from build123d import *

# Parameters (mm, degrees)
BOSS_EXTRUDE1_DEPTH = 10
CUT_EXTRUDE1_DEPTH  = 42.158231255
FILLET1_R           = 3
BOSS_EXTRUDE2_DEPTH = 3.5
SKETCH4_W           = 8
SKETCH4_H           = 2.5
BOSS_EXTRUDE3_DEPTH = 5
CIRPATTERN1_COUNT   = 2
CIRPATTERN1_ANGLE   = 180


with BuildPart() as part:
    # Sketch1 → Boss-Extrude1 (new, symmetric)
    with BuildSketch(Plane(origin=(0, 0, 0), x_dir=(1, 0, 0), z_dir=(0, 1, 0))):
        with BuildLine():
            Line((-9, 0), (9.75, 0))
            ThreePointArc((9.75, 0), (13.639087297, -1.610912703), (15.25, -5.5))
            Line((15.25, -5.5), (15.25, -9.5))
            ThreePointArc((15.25, -9.5), (16.128679656, -11.621320344), (18.25, -12.5))
            Line((18.25, -12.5), (37, -12.5))
            Line((37, -12.5), (37, -15))
            Line((37, -15), (18.25, -15))
            ThreePointArc((18.25, -15), (14.360912703, -13.389087297), (12.75, -9.5))
            Line((12.75, -9.5), (12.75, -5.5))
            ThreePointArc((12.75, -5.5), (11.871320344, -3.378679656), (9.75, -2.5))
            Line((9.75, -2.5), (-9, -2.5))
            Line((-9, -2.5), (-9, 0))
        make_face()
    extrude(amount=BOSS_EXTRUDE1_DEPTH, both=True)

    # Sketch2 → Cut-Extrude1 (cut, through all)
    with BuildSketch(Plane.XY):
        with BuildLine():
            Line((-2.75, 0), (-2.75, -10))
            Line((-2.75, -10), (2.75, -10))
            Line((2.75, -10), (2.75, 0))
            ThreePointArc((2.75, 0), (0, 2.75), (-2.75, 0))
        make_face()
        with BuildLine():
            Line((25.25, 0), (25.25, -10))
            Line((25.25, -10), (30.75, -10))
            Line((30.75, -10), (30.75, 0))
            ThreePointArc((30.75, 0), (28, 2.75), (25.25, 0))
        make_face()
    extrude(amount=CUT_EXTRUDE1_DEPTH, mode=Mode.SUBTRACT)

    # Fillet1
    fillet1_edges = [part.edges().sort_by_distance(p)[0] for p in [
        (37, -10, 13.75),
        (-9, -10, 1.25),
        (37, 10, 13.75),
        (2.75, -10, 1.25),
        (-2.75, -10, 1.25),
        (-9, 10, 1.25),
        (25.25, -10, 13.75),
        (30.75, -10, 13.75),
    ]]
    fillet(fillet1_edges, radius=FILLET1_R)

    # Sketch3 → Boss-Extrude2 (add)
    with BuildSketch(Plane.XY.offset(2.5)):
        Polygon((0, 4.618802154), (-4, 2.309401077), (-4, -2.309401077), (0, -4.618802154), (4, -2.309401077), (4, 2.309401077), align=None)
    boss_extrude2 = extrude(amount=BOSS_EXTRUDE2_DEPTH)

    # Sketch4 → Revolve1 (revolve)
    with BuildSketch(Plane(origin=(0, 0, 0), x_dir=(0, 0, -1), z_dir=(1, 0, 0))):
        with Locations((1.5, 1.25)):
            Rectangle(SKETCH4_W, SKETCH4_H)
    revolve1 = revolve(axis=Axis((0, 0, -5.5), (0, 0, 1)))

    # Sketch5 → Cut-Revolve1 (revolve, cut)
    with BuildSketch(Plane(origin=(0, 0, 0), x_dir=(0, 0, -1), z_dir=(1, 0, 0))):
        Polygon((-2.5, 4.618802154), (-2.5, 4), (-2.85726559, 4.618802154), align=None)
        Polygon((-5.64273441, 4.618802154), (-6, 4.618802154), (-6, 4), align=None)
    cut_revolve1 = revolve(axis=Axis((0, 0, 2.5), (0, 0, 1)), mode=Mode.SUBTRACT)

    # Sketch6 → Boss-Extrude3 (add, symmetric)
    with BuildSketch(Plane(origin=(0, 0, 0), x_dir=(0, 0, -1), z_dir=(1, 0, 0))):
        with BuildLine():
            Line((5.172072931, 2.989575498), (2.36192258, 4.957263957))
            ThreePointArc((2.36192258, 4.957263957), (2.123797819, 4.972871479), (2, 4.768858987))
            Line((2, 4.768858987), (2, 2.9))
            Line((2, 2.9), (1.4, 2.9))
            ThreePointArc((1.4, 2.9), (1.258578644, 2.841421356), (1.2, 2.7))
            Line((1.2, 2.7), (1.2, -2.7))
            ThreePointArc((1.2, -2.7), (1.258578644, -2.841421356), (1.4, -2.9))
            Line((1.4, -2.9), (2, -2.9))
            Line((2, -2.9), (2, -4.768858987))
            ThreePointArc((2, -4.768858987), (2.123797819, -4.972871479), (2.36192258, -4.957263957))
            Line((2.36192258, -4.957263957), (5.172072931, -2.989575498))
            ThreePointArc((5.172072931, -2.989575498), (5.26610325, -2.882354469), (5.3, -2.743829885))
            Line((5.3, -2.743829885), (5.3, 2.743829885))
            ThreePointArc((5.3, 2.743829885), (5.26610325, 2.882354469), (5.172072931, 2.989575498))
        make_face()
    boss_extrude3 = extrude(amount=BOSS_EXTRUDE3_DEPTH, both=True)

    # CirPattern1: Boss-Extrude2, Revolve1, Cut-Revolve1, Boss-Extrude3 ×2 about axis
    cirpattern1_axis = Axis((14, 11, 7.5), (0, -1, 0))
    add([boss_extrude2.rotate(cirpattern1_axis, i * CIRPATTERN1_ANGLE / (CIRPATTERN1_COUNT - 1)) for i in range(1, CIRPATTERN1_COUNT)])
    add([revolve1.rotate(cirpattern1_axis, i * CIRPATTERN1_ANGLE / (CIRPATTERN1_COUNT - 1)) for i in range(1, CIRPATTERN1_COUNT)])
    add([cut_revolve1.rotate(cirpattern1_axis, i * CIRPATTERN1_ANGLE / (CIRPATTERN1_COUNT - 1)) for i in range(1, CIRPATTERN1_COUNT)], mode=Mode.SUBTRACT)
    add([boss_extrude3.rotate(cirpattern1_axis, i * CIRPATTERN1_ANGLE / (CIRPATTERN1_COUNT - 1)) for i in range(1, CIRPATTERN1_COUNT)])


solid = part.part
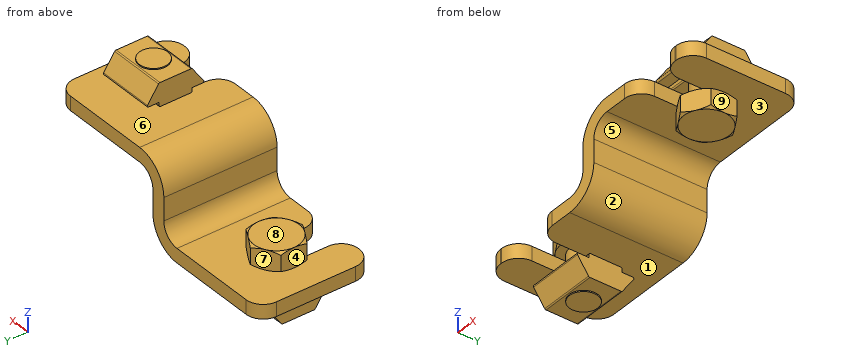
Design review of the part built by this model. Coordinates are the model's own, in mm. Face numbers are marked on the shaded views. A direction names the side the tool comes from. Give positions to 0.01 mm unless a question says otherwise; leave off trailing zeros. Order: outer loops, then holes, each group sorted by start corner. A loop starts at its lowest first (then second) coordinate and runs counter-clockwise, first axis right, second up. Notation, with made-up numbers: (-16, 88.5) - (42, 88.5) arc R32 ccw to (42, 124.5) - close; hole circle Ø2 at (88.25, -14.5). An arc over 180 degrees is marked (long way). Use CSV: the item, a comma, the result in double quotes. Start each with the question number.
Q1. Take a section at A-A (z = 11.5). State the section outline as (x, y) points.
Q2. Machinability: for the marked faces 5, 6, 7, 8 and 9, which of the approach directions +Z, -Z, +X, -X, +Y, -Y give a long, thin tool a straight path to every point of the face, cutting with its end or side? Answer none if there is none.
Q3. Draft analysis for pull direction X (two halves, no side actions). For the marked faces 1, 2, 3 and 4, state which applies: pulls with the +X half, pulls with the -X half, needs draft (parallel to the pull), parting line crosses it, or undercut.
Q4. For P1, Ø3, axis at y = -4.5, z = 7.5, coming from the +X side; P2, Ø1.5, axis at x = 12, z = -1.5, coming from the +Y side (3 decimals); P3, Ø3, axis at y = -1, z = 10.5, coming from the -X side; P4, Ø4.5, axis at x = 27, y = -0.5, coming from the -Z side, all flat-tipped, find the tip position at first contact; note any pin that passes through.
Q5. Take a section at D-D (y = 8.5). State the section outline as (x, z) points, and give its area (3 significant figures).
Q6. Take a section at C-C (z = 1.5). State the section outline as (x, y) points.
Q7. For line 1 (X direction, y = 1, z = 9.5); line 2 (Z direction, x = 32.5, y = 2.75); line 3 (Z direction, x = 20.5, y = -5.25), list the stretches that pass through material, from the lowest coordinate up.
Q8. Take a section at B-B (y = -8.25). State the section outline as (x, z) points, and give its area (3 significant figures).
Calculated:
1,outline,"(13.13, -10) - (16.01, -10) - (16.01, 10) - (13.13, 10) - close; (24, -2.31) - (28, -4.62) - (32, -2.31) - (32, 2.31) - (28, 4.62) - (24, 2.31) - close"
2,face 5,"-Z, +Y, -Y"
2,face 6,"+Y"
2,face 7,"+Z, -X, +Y"
2,face 8,"+Z, -X, +Y, -Y"
2,face 9,"-Z, +X, +Y, -Y"
3,face 1,"needs draft"
3,face 2,"pulls with the +X half"
3,face 3,"undercut"
3,face 4,"pulls with the -X half"
4,P1,"stops at x = 15.25"
4,P2,"passes through"
4,P3,"stops at x = 12.75"
4,P4,"stops at z = 9"
5,outline,"(-8.6, 0) - (9.75, 0) arc R5.5 ccw to (15.25, 5.5) - (15.25, 9.5) arc R3 cw to (18.25, 12.5) - (36.6, 12.5) - (36.6, 15) - (18.25, 15) arc R5.5 ccw to (12.75, 9.5) - (12.75, 5.5) arc R3 cw to (9.75, 2.5) - (-8.6, 2.5) - close"
5,area,"135 mm²"
6,outline,"(-9, -7) arc R3 ccw to (-6, -10) - (-5.75, -10) arc R3 ccw to (-2.75, -7) - (-2.75, 0) arc R2.75 cw to (2.75, 0) - (2.75, -7) arc R3 ccw to (5.75, -10) - (13.52, -10) - (13.52, 10) - (-6, 10) arc R3 ccw to (-9, 7) - close; circle Ø5 at (0, 0)"
7,line 1,"x = 12.75 to 15.25, 24 to 32"
7,line 2,"z = 12.5 to 15, 16.21 to 20.3"
7,line 3,"z = 12.5 to 15"
8,outline,"(-8.73, 0) - (-3.02, 0) - (-3.02, 2.5) - (-8.73, 2.5) - close; (3.02, 0) - (9.75, 0) arc R5.5 ccw to (15.25, 5.5) - (15.25, 9.5) arc R3 cw to (18.25, 12.5) - (24.98, 12.5) - (24.98, 15) - (18.25, 15) arc R5.5 ccw to (12.75, 9.5) - (12.75, 5.5) arc R3 cw to (9.75, 2.5) - (3.02, 2.5) - close; (31.02, 12.5) - (36.73, 12.5) - (36.73, 15) - (31.02, 15) - close"
8,area,"106 mm²"
